Input: part model. Units: mm. Frame: model coordinates. A direction names the side the tool comes from. Give positions to 0.01 mm unless a question says otherwise; leave off trailing zeros. Loops run counter-clockwise (first coordinate to the right, second up) from the corner with the lowest first, then second, coordinate; pieces in that order, holes last.
from build123d import *

# Parameters (mm, degrees)
BOSS_EXTRUDE1_DEPTH      = 3
SKETCH2_W                = 27.727272727
SKETCH2_H                = 3
SKETCH2_W_2              = 3
SKETCH2_H_2              = 18
SKETCH2_H_3              = 9
SKETCH2_W_3              = 23.343342349
SKETCH2_W_4              = 23.34334235
SKETCH2_W_5              = 6
CUT_EXTRUDE1_DEPTH       = 157.058482628
CUT_EXTRUDE1_DEPTH_BACK  = 157.058482628
SKETCH3_W                = 3.2
SKETCH3_H                = 10.5
SKETCH3_W_2              = 5.2
SKETCH3_H_2              = 2.5
CUT_EXTRUDE2_DEPTH       = 157.058482628
CUT_EXTRUDE2_DEPTH_BACK  = 157.058482628
FILLET1_R                = 2.5
BOSS_EXTRUDE2_DEPTH      = 3
FILLET2_R                = 2.5
SKETCH6_R                = 5
SKETCH6_R_2              = 1.65
CUT_EXTRUDE5_DEPTH       = 250.147044935
CUT_EXTRUDE5_DEPTH_BACK  = 250.147044935
SKETCH8_R                = 10
CUT_EXTRUDE6_DEPTH       = 250.147044935
CUT_EXTRUDE6_DEPTH_BACK  = 250.147044935
SKETCH9_W                = 20
SKETCH9_H                = 3
CUT_EXTRUDE7_DEPTH       = 250.147044935
CUT_EXTRUDE7_DEPTH_BACK  = 250.147044935
SKETCH10_W               = 23.343342349
SKETCH10_H               = 3
SKETCH10_R               = 10
SKETCH10_W_2             = 23.34334235
CUT_EXTRUDE8_DEPTH       = 250.147044935
CUT_EXTRUDE8_DEPTH_BACK  = 250.147044935
SKETCH11_W               = 27.840909091
SKETCH11_H               = 3
CUT_EXTRUDE9_DEPTH       = 250.147044935
CUT_EXTRUDE9_DEPTH_BACK  = 250.147044935
FILLET3_R                = 5
SKETCH12_W               = 5
SKETCH12_H               = 12
CUT_EXTRUDE10_DEPTH      = 250.147044935
CUT_EXTRUDE10_DEPTH_BACK = 250.147044935


with BuildPart() as part:
    # Sketch1 → Boss-Extrude1 (new body)
    with BuildSketch(Plane(origin=(0, 0, 0), x_dir=(0, 0, -1), z_dir=(1, 0, 0))):
        with BuildLine():
            Line((-152.5, 33), (152.5, 33))
            Line((152.5, 33), (152.5, 23))
            Line((152.5, 23), (107.5, 23))
            ThreePointArc((107.5, 23), (72.144660941, 8.355339059), (57.5, -27))
            Line((57.5, -27), (57.5, -33))
            Line((57.5, -33), (-152.5, -33))
            Line((-152.5, -33), (-152.5, 33))
        make_face()
    extrude(amount=BOSS_EXTRUDE1_DEPTH)

    # Sketch2 → Cut-Extrude1 (cut, two sides)
    with BuildSketch(Plane(origin=(3, 0, 0), x_dir=(0, 0, -1), z_dir=(1, 0, 0))) as cut_extrude1_sk:
        with Locations((-138.636363636, 31.5)):
            Rectangle(SKETCH2_W, SKETCH2_H)
        with Locations((-83.181818182, 31.5)):
            Rectangle(SKETCH2_W, SKETCH2_H)
        with Locations((-27.727272728, 31.5)):
            Rectangle(SKETCH2_W, SKETCH2_H)
        with Locations((-151, 3)):
            Rectangle(SKETCH2_W_2, SKETCH2_H_2)
        with Locations((-151, -28.5)):
            Rectangle(SKETCH2_W_2, SKETCH2_H_3)
        with Locations((-117.484986475, -28.5)):
            Rectangle(SKETCH2_W_3, SKETCH2_H)
        with Locations((-70.798301777, -28.5)):
            Rectangle(SKETCH2_W_3, SKETCH2_H)
        with Locations((22.575067622, -28.5)):
            Rectangle(SKETCH2_W_4, SKETCH2_H)
        with Locations((149.5, 31.5)):
            Rectangle(SKETCH2_W_5, SKETCH2_H)
        with Locations((-24.111617078, -28.5)):
            Rectangle(SKETCH2_W_3, SKETCH2_H)
    extrude(amount=CUT_EXTRUDE1_DEPTH, mode=Mode.SUBTRACT)
    extrude(cut_extrude1_sk.sketch, amount=-CUT_EXTRUDE1_DEPTH_BACK, mode=Mode.SUBTRACT)

    # Sketch3 → Cut-Extrude2 (cut, two sides)
    with BuildSketch(Plane(origin=(3, 0, 0), x_dir=(0, 0, -1), z_dir=(1, 0, 0))) as cut_extrude2_sk:
        with Locations((-110.909090909, 27.75)):
            Rectangle(SKETCH3_W, SKETCH3_H)
        with Locations((-110.909090909, 28.575)):
            Rectangle(SKETCH3_W_2, SKETCH3_H_2)
    extrude(amount=CUT_EXTRUDE2_DEPTH, mode=Mode.SUBTRACT)
    extrude(cut_extrude2_sk.sketch, amount=-CUT_EXTRUDE2_DEPTH_BACK, mode=Mode.SUBTRACT)

    # Fillet1
    fillet1_edges = [part.edges().sort_by_distance(p)[0] for p in [
        (1.5, -33, -57.5),
    ]]
    fillet(fillet1_edges, radius=FILLET1_R)

    # Sketch4 → Boss-Extrude2 (add)
    with BuildSketch(Plane(origin=(0, 0, 0), x_dir=(0, 0, -1), z_dir=(1, 0, 0))):
        with BuildLine():
            Line((-83.181818182, 33), (-83.181818182, 30))
            Line((-83.181818182, 30), (35.818181818, 30))
            Line((35.818181818, 30), (35.818181818, 33))
            Line((35.818181818, 33), (25.753026775, 61.931534749))
            Line((25.753026775, 61.931534749), (59.886459158, 33))
            Line((59.886459158, 33), (90.818181818, 33))
            Line((90.818181818, 33), (12.817635516, 99.113348651))
            Line((12.817635516, 99.113348651), (-16.565017269, 183.571584658))
            ThreePointArc((-16.565017269, 183.571584658), (-36.922973482, 196.946020133), (-55.102803407, 180.73442893))
            Line((-55.102803407, 180.73442893), (-83.181818182, 33))
        make_face()
        Polygon((6.913219914, 40), (-46.974972009, 40), (-3.929894771, 71.167721507), align=None, mode=Mode.SUBTRACT)
        Polygon((-54.643252411, 49.263022537), (-34.033564648, 157.698467174), (-8.047004759, 83.002045982), align=None, mode=Mode.SUBTRACT)
    extrude(amount=BOSS_EXTRUDE2_DEPTH)

    # Fillet2
    fillet2_edges = [part.edges().sort_by_distance(p)[0] for p in [
        (1.5, 33, -59.886459158),
        (1.5, 61.931534749, -25.753026775),
        (1.5, 33, -35.818181818),
        (1.5, 40, -6.913219914),
        (1.5, 71.167721507, 3.929894771),
        (1.5, 40, 46.974972009),
        (1.5, 49.263022537, 54.643252411),
        (1.5, 83.002045982, 8.047004759),
        (1.5, 157.698467174, 34.033564648),
    ]]
    fillet(fillet2_edges, radius=FILLET2_R)

    # Sketch6 → Cut-Extrude5 (cut, two sides)
    with BuildSketch(Plane(origin=(3, 0, 0), x_dir=(0, 0, -1), z_dir=(1, 0, 0))) as cut_extrude5_sk:
        with Locations((-35.454545455, 177)):
            Circle(SKETCH6_R)
        with Locations((-1.492946709, 95.333591431)):
            Circle(SKETCH6_R_2)
        with Locations((27.342535354, 25.993797473)):
            Circle(SKETCH6_R_2)
    extrude(amount=CUT_EXTRUDE5_DEPTH, mode=Mode.SUBTRACT)
    extrude(cut_extrude5_sk.sketch, amount=-CUT_EXTRUDE5_DEPTH_BACK, mode=Mode.SUBTRACT)

    # Sketch8 → Cut-Extrude6 (cut, two sides)
    with BuildSketch(Plane(origin=(0, 0, 0), x_dir=(0, 0, -1), z_dir=(1, 0, 0))) as cut_extrude6_sk:
        with Locations((-5, 0)):
            Circle(SKETCH8_R)
        with Locations((-40, 0)):
            Circle(SKETCH8_R)
    extrude(amount=CUT_EXTRUDE6_DEPTH, mode=Mode.SUBTRACT)
    extrude(cut_extrude6_sk.sketch, amount=-CUT_EXTRUDE6_DEPTH_BACK, mode=Mode.SUBTRACT)

    # Sketch9 → Cut-Extrude7 (cut, two sides)
    with BuildSketch(Plane(origin=(0, 0, 0), x_dir=(0, 0, -1), z_dir=(1, 0, 0))) as cut_extrude7_sk:
        Polygon((-68.111670983, 53.378521315), (-64.377242053, 73.026779267), (-61.43000336, 72.466614928), (-65.16443229, 52.818356975), align=None)
        Polygon((-55.507973344, 119.691391905), (-52.707151647, 134.427585369), (-49.759912954, 133.867421029), (-52.560734651, 119.131227565), align=None)
        Polygon((64.311409407, 40.391956194), (49.054577079, 53.32366402), (50.994333253, 55.612188869), (66.251165581, 42.680481043), align=None)
        with Locations((-17.931502251, 33)):
            Rectangle(SKETCH9_W, SKETCH9_H)
    extrude(amount=CUT_EXTRUDE7_DEPTH, mode=Mode.SUBTRACT)
    extrude(cut_extrude7_sk.sketch, amount=-CUT_EXTRUDE7_DEPTH_BACK, mode=Mode.SUBTRACT)

    # Sketch10 → Cut-Extrude8 (cut, two sides)
    with BuildSketch(Plane(origin=(0, 0, 0), x_dir=(0, 0, -1), z_dir=(1, 0, 0))) as cut_extrude8_sk:
        with BuildLine():
            Line((-149.5, -33), (55, -33))
            ThreePointArc((55, -33), (56.767766953, -32.267766953), (57.5, -30.5))
            Line((57.5, -30.5), (57.5, -27))
            ThreePointArc((57.5, -27), (71.867312479, 8.075797639), (106.712463201, 22.993797473))
            Line((106.712463201, 22.993797473), (39.832195251, 22.993797473))
            Line((39.832195251, 22.993797473), (34.842535354, 19.5))
            Line((34.842535354, 19.5), (19.842535354, 19.5))
            Line((19.842535354, 19.5), (14.852875457, 22.993797473))
            Line((14.852875457, 22.993797473), (-64.61787351, 22.993797473))
            Line((-64.61787351, 22.993797473), (-68.111670983, 19.5))
            Line((-68.111670983, 19.5), (-95.196498882, 19.5))
            Line((-95.196498882, 19.5), (-100.909090909, 15.5))
            Line((-100.909090909, 15.5), (-120.909090909, 15.5))
            Line((-120.909090909, 15.5), (-126.621682936, 19.5))
            Line((-126.621682936, 19.5), (-152.5, 19.5))
            Line((-152.5, 19.5), (-152.5, 12))
            Line((-152.5, 12), (-149.5, 12))
            Line((-149.5, 12), (-149.5, -6))
            Line((-149.5, -6), (-152.5, -6))
            Line((-152.5, -6), (-152.5, -24))
            Line((-152.5, -24), (-149.5, -24))
            Line((-149.5, -24), (-149.5, -33))
        make_face()
        with Locations((-117.484986475, -28.5)):
            Rectangle(SKETCH10_W, SKETCH10_H, mode=Mode.SUBTRACT)
        with Locations((-70.798301777, -28.5)):
            Rectangle(SKETCH10_W, SKETCH10_H, mode=Mode.SUBTRACT)
        with Locations((-24.111617078, -28.5)):
            Rectangle(SKETCH10_W, SKETCH10_H, mode=Mode.SUBTRACT)
        with Locations((-40, 0)):
            Circle(SKETCH10_R, mode=Mode.SUBTRACT)
        with Locations((-5, 0)):
            Circle(SKETCH10_R, mode=Mode.SUBTRACT)
        with Locations((22.575067622, -28.5)):
            Rectangle(SKETCH10_W_2, SKETCH10_H, mode=Mode.SUBTRACT)
    extrude(amount=CUT_EXTRUDE8_DEPTH, mode=Mode.SUBTRACT)
    extrude(cut_extrude8_sk.sketch, amount=-CUT_EXTRUDE8_DEPTH_BACK, mode=Mode.SUBTRACT)

    # Sketch11 → Cut-Extrude9 (cut, two sides)
    with BuildSketch(Plane(origin=(0, 0, 0), x_dir=(0, 0, -1), z_dir=(1, 0, 0))) as cut_extrude9_sk:
        with Locations((104.738636364, 31.5)):
            Rectangle(SKETCH11_W, SKETCH11_H)
    extrude(amount=CUT_EXTRUDE9_DEPTH, mode=Mode.SUBTRACT)
    extrude(cut_extrude9_sk.sketch, amount=-CUT_EXTRUDE9_DEPTH_BACK, mode=Mode.SUBTRACT)

    # Fillet3
    fillet3_edges = [part.edges().sort_by_distance(p)[0] for p in [
        (1.5, 15.5, 100.909090909),
        (1.5, 19.5, 95.196498882),
        (1.5, 19.5, 68.111670983),
        (1.5, 22.993797473, 64.61787351),
        (1.5, 22.993797473, -14.852875457),
        (1.5, 19.5, -19.842535354),
        (1.5, 19.5, -34.842535354),
        (1.5, 22.993797473, -39.832195251),
        (1.5, 19.5, 126.621682936),
        (1.5, 15.5, 120.909090909),
    ]]
    fillet(fillet3_edges, radius=FILLET3_R)

    # Sketch12 → Cut-Extrude10 (cut, two sides)
    with BuildSketch(Plane(origin=(3, 0, 0), x_dir=(0, 0, -1), z_dir=(1, 0, 0))) as cut_extrude10_sk:
        with Locations((-35.454545455, 161.5)):
            Rectangle(SKETCH12_W, SKETCH12_H)
    extrude(amount=CUT_EXTRUDE10_DEPTH, mode=Mode.SUBTRACT)
    extrude(cut_extrude10_sk.sketch, amount=-CUT_EXTRUDE10_DEPTH_BACK, mode=Mode.SUBTRACT)


solid = part.part
(1) Mould query, pull axis Y, two halves, no side actions, for faces 3 (the flat face through (1.479, 67.635, 29.269)), 4 (the flat face through (1.479, 140.751, 1.668)), 5 (the flat face through (3, 79.8, 12)), 6 (the flat face through (1.479, 101.329, 44.747)). Classes: +Y half, -Y half, draft (parallel to the pull), parting line (faces both ways), or undercut.
Values follow:
face 3: undercut
face 4: +Y half
face 5: draft
face 6: undercut
(2) Cut plane C-C (x = 1). Count the separate pieces of the cut face and the enclosed holes in it, and give its area (3 significant figures).
Values follow:
separate pieces: 1
enclosed holes: 11
area: 13,600 mm2
(3) Ray query, probe 1 along Z at (x, y) = (1.5, 124); probe 2 along Z at (x, y) = (1.2, 65); probe 3 along Z at (x, y) = (0.5, 68). Return the intervals inside material, ascending.
Values follow:
probe 1: z = -4.16 to 22.31, 40.44 to 51.64, 54.69 to 65.89
probe 2: z = -53.06 to 1.78, 12.45 to 32.91, 51.65 to 62.85, 65.9 to 77.1
probe 3: z = -49.53 to 2.83, 8.3 to 28.77, 51.08 to 62.28, 65.33 to 76.53
(4) Pin query (flat end, axial travel): pin 1 Ø1 at (x, z) = (1.5, 30.5) entering from -Y; pin 2 Ø0.9 at (x, z) = (1, 92.5) entering from +Y; pin 3 Ø1.1 at (x, z) = (2, 108.5) entering from +Y. Return the tip coordinate at first contact, or that it passes through.
Values follow:
pin 1: stops at y = 22.99
pin 2: stops at y = 30
pin 3: stops at y = 33
(5) Reachability of faces 1 (the flat face through (1.479, 55.83, -1.406)), 2 (the flat face through (0, 79.8, 12)) from +Z, -Z, +X, -X, +Y, -Y: full face, straight path, thin tool, end or side. Return the list, or none.
Values follow:
face 1: +X, -X
face 2: +Z, -Z, -X, +Y, -Y
(6) Cut plane A-A (y = 177). Return the cut outline in (x, z).
Values follow:
outline: (0, 14.28) - (3, 14.28) - (3, 30.45) - (0, 30.45) - close; (0, 40.45) - (3, 40.45) - (3, 55.81) - (0, 55.81) - close
(7) Cut plane B-B (y = 60.5). Return the cut outline in (x, z), and give its area (3 significant figures).
Values follow:
outline: (0, -58.37) - (3, -58.37) - (3, 0.22) - (0, 0.22) - close; (0, 18.66) - (3, 18.66) - (3, 39.12) - (0, 39.12) - close; (0, 52.51) - (3, 52.51) - (3, 63.7) - (0, 63.7) - close; (0, 66.76) - (3, 66.76) - (3, 77.96) - (0, 77.96) - close
area: 304 mm2
(8) Cut plane D-D (y = 103). Return the cut outline in (x, z).
Values follow:
outline: (0, -11.47) - (3, -11.47) - (3, 15) - (0, 15) - close; (0, 44.43) - (3, 44.43) - (3, 69.88) - (0, 69.88) - close
